The figure shows three views and two pictorial views of one solid part (mm, origin at its lowest corner). Answer the questions. A direction names the side the tool comes from. Coordinates: 2 decimals unless noted, no trailing zeros. Order: outer loops, then holes, each group sorted by start corner. A loop starts at its lowest first (then second) coordinate and runs counter-clockwise, first axis right, second up. Notation, with made-up numbers: M 50,-33.5 L 90,-33.5 A19 ccw 90,-24.5 Z; hole C -18.5,52.25 d2. An arc over 180 degrees is marked long. Use a Markdown table: item, result.
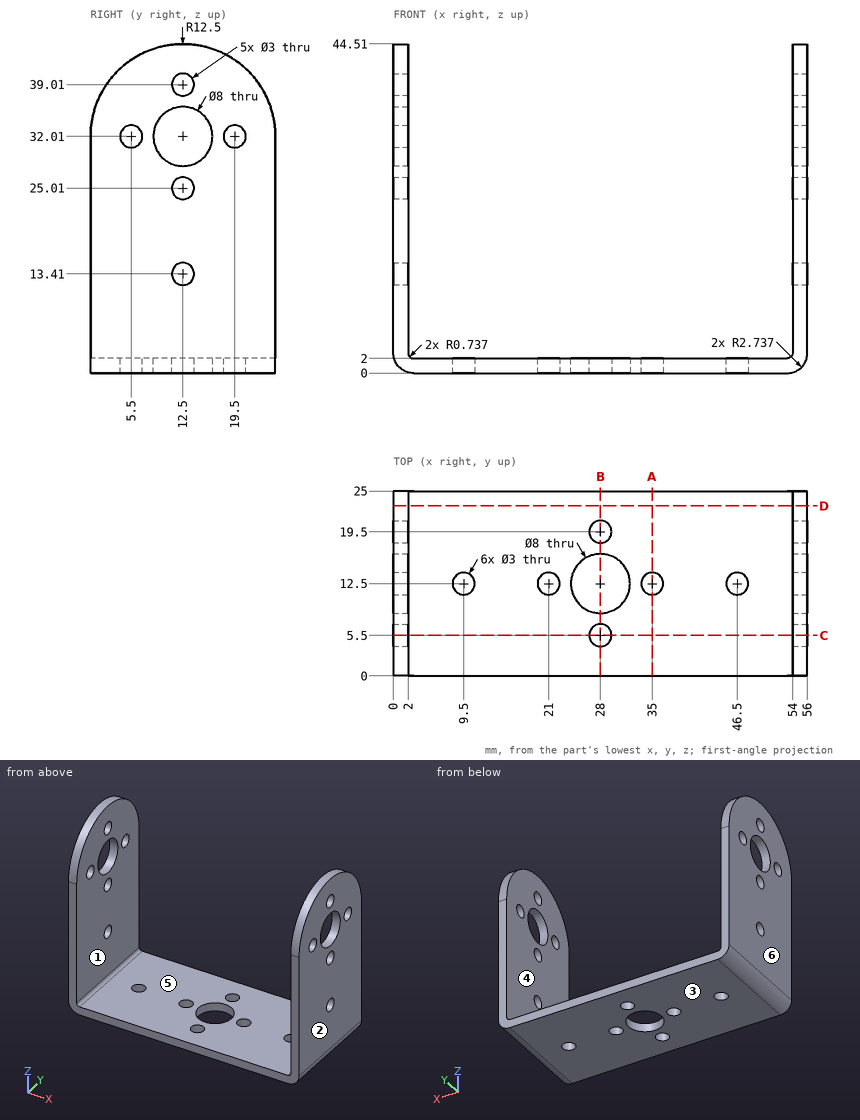
1. Section C-C on y = 5.5 is taken. Determine the outline of the cut face in (x, z).
Answers below:
| item | result |
|---|---|
| outline | M 0,2.74 A2.74 ccw 2.74,0 L 26.5,0 L 26.5,2 L 2.74,2 A0.74 cw 2,2.74 L 2,30.51 L 0,30.51 Z; M 0,33.51 L 2,33.51 L 2,42.37 L 0,42.37 Z; M 29.5,0 L 53.26,0 A2.74 ccw 56,2.74 L 56,30.51 L 54,30.51 L 54,2.74 A0.74 cw 53.26,2 L 29.5,2 Z; M 54,33.51 L 56,33.51 L 56,42.37 L 54,42.37 Z |
2. A flat-ended cylindrical pin translates along its axis: P1, Ø3, axis at x = 25, y = 22, coming from the +Z side. Find the tip coordinate at first contact, or state that the pin passes through.
Answers below:
| item | result |
|---|---|
| P1 | z = 2 |
3. Find the intervals of material crossed by probe 1 along Y at (x, z) = (28, 1.1); probe 2 along X at (y, z) = (17, 8.5); probe 3 along Z at (x, y) = (23.5, 2.5), in increasing order.
Answers below:
| item | result |
|---|---|
| probe 1 | 0 to 4, 7 to 8.5, 16.5 to 18, 21 to 25 |
| probe 2 | 0 to 2, 54 to 56 |
| probe 3 | 0 to 2 |
4. Section D-D on y = 23 is taken. Determine the outline of the cut face in (x, z).
Answers below:
| item | result |
|---|---|
| outline | M 0,2.74 A2.74 ccw 2.74,0 L 53.26,0 A2.74 ccw 56,2.74 L 56,38.79 L 54,38.79 L 54,2.74 A0.74 cw 53.26,2 L 2.74,2 A0.74 cw 2,2.74 L 2,38.79 L 0,38.79 Z |
5. Section A-A on x = 35 is taken. Determine the outline of the cut face in (y, z).
Answers below:
| item | result |
|---|---|
| outline | M 0,0 L 11,0 L 11,2 L 0,2 Z; M 14,0 L 25,0 L 25,2 L 14,2 Z |
6. For the marked faces 1 and 2, determine the directions among +Z, -Z, +X, -X, +Y, -Y from which every point of the face is accessible in a straight line to the end or side of a thin tool.
Answers below:
| item | result |
|---|---|
| face 1 | +Z, +Y, -Y |
| face 2 | +Z, -Z, +X, +Y, -Y |
7. Section B-B on x = 28 is taken. Determine the outline of the cut face in (y, z).
Answers below:
| item | result |
|---|---|
| outline | M 0,0 L 4,0 L 4,2 L 0,2 Z; M 7,0 L 8.5,0 L 8.5,2 L 7,2 Z; M 16.5,0 L 18,0 L 18,2 L 16.5,2 Z; M 21,0 L 25,0 L 25,2 L 21,2 Z |
8. For a pull along X with two mould halves and no side action, classify the marked faces 3, 4, 5 and 6 as +X half, -X half, draft (parallel to the pull), parting line (faces both ways), or undercut.
Answers below:
| item | result |
|---|---|
| face 3 | draft |
| face 4 | undercut |
| face 5 | undercut |
| face 6 | -X half |
